Read the model definition and answer for the solid it produces. Units are mm, in the model's axes. A direction names the side the tool comes from. Coordinates: 2 decimals unless noted, no trailing zeros. Order: outer loops, then holes, each group sorted by start corner. A loop starts at its lowest first (then second) coordinate and runs counter-clockwise, first axis right, second up.
Autodesk Inventor part; units mm, degrees
ref_plane "YZ Plane" through (0, 0, 0) normal (1, 0, 0) x (0, 1, 0)
ref_plane "XZ Plane" through (0, 0, 0) normal (0, 1, 0) x (-1, 0, 0)
ref_plane "XY Plane" through (0, 0, 0) normal (0, 0, 1) x (1, 0, 0)
sketch "Sketch1" plane through (0, 0, 0) normal (1, 0, 0) x (0, 1, 0)
  line L0 (0, 0) -> (24, 0)
  line L1 (24, 0) -> (0, 89.5692)
  line L2 (0, 89.5692) -> (0, 0)
  line L3 (24, 0) -> (30, 0)
  line L4 (7.8518, 60.2659) -> (13.6473, 61.8188)
  line L5 (30, 0) -> (0, 113.0916)
  line L6 (0, 113.0916) -> (0, 89.5692)
  point P0 (0, 23.8051)
  point P1 (17.3305, 0)
  point P2 (0, 30.632)
  dimension "d0" = 24
  dimension "d1" = 75
  dimension "d2" = 6
  dimension "d3" = 6
  dimension "d4" = 90
extrude "Extrusion1" add sketch "Sketch1" along normal blind 40
sketch "Sketch5" plane through (0, 0, 0) normal (0, 0, -1) x (-1, 0, 0)
  line L0 (0, 0) -> (0, 30)
  line L1 (-40, 0) -> (-4, 0)
  line L2 (-4, 0) -> (-4, 14)
  line L3 (-4, 14) -> (-40, 14)
  line L4 (-40, 14) -> (-40, 0)
  point P0 (0, 18)
  dimension "d24" = 36
  dimension "d25" = 14
extrude "Extrusion2" cut sketch "Sketch5" against normal blind 52.575
sketch "Sketch7" plane through (4, 14, 0) normal (0, -1, 0) x (1, 0, 0)
  line L0 (0, 0) -> (0, 52.575)
  line L1 (36, 52.575) -> (0, 0)
  line L2 (0, 0) -> (0, 3.8616)
  line L3 (0, 3.8616) -> (33.3558, 52.575)
  line L4 (36, 52.575) -> (0, 52.575)
  line L5 (33.3558, 52.575) -> (36, 52.575)
  point P0 (-4, 0)
extrude "Extrusion4" add sketch "Sketch7" along normal blind 14 contours L0 L3 L4 L1
sketch "Sketch8" plane through (0, 0, 0) normal (0, -1, 0) x (1, 0, 0)
  line L0 (36.9948, 58.9837) -> (3.2686, 58.9837)
  line L1 (3.2686, 58.9837) -> (3.2686, 93.3042)
  line L2 (3.2686, 93.3042) -> (36.9948, 93.3042)
  line L3 (36.9948, 93.3042) -> (36.9948, 58.9837)
  point P0 (0, 0)
extrude "Extrusion5" cut sketch "Sketch8" against normal blind 3.4625
sketch "Sketch9" plane through (0, 3.4625, 0) normal (0, -1, 0) x (1, 0, 0)
  line L0 (36.9948, 58.9837) -> (3.2686, 58.9837)
  line L1 (3.2686, 58.9837) -> (3.2686, 93.3042)
  line L2 (36.9948, 58.9837) -> (3.2686, 58.9837)
  line L3 (3.2686, 58.9837) -> (3.2686, 72.9495)
  line L4 (3.2686, 72.9495) -> (36.9948, 72.9495)
  line L5 (36.9948, 72.9495) -> (36.9948, 58.9837)
  point P0 (0, 0)
extrude "Extrusion6" cut sketch "Sketch9" against normal blind 6.0625
sketch "Sketch10" plane through (0, 0, 0) normal (0, 0, -1) x (-1, 0, 0)
  line L0 (-40, 30) -> (-40, 0)
  line L1 (0, 30) -> (0, 0)
  line L2 (-40, 27) -> (0, 27)
  line L3 (0, 27) -> (0, 21)
  line L4 (0, 21) -> (-40, 21)
  line L5 (-40, 21) -> (-40, 27)
  line L6 (0, 30) -> (-40, 30)
  dimension "d35" = 6
  dimension "d36" = 3
extrude "Extrusion7" add sketch "Sketch10" along normal blind 6 contours L2 L1 L4 L0
properties part number "RAMP"
1) Flat-ended cylindrical pins translate along their axes: pin 1 Ø18 at (x, z) = (21.5, 34) entering from -Y; pin 2 Ø2.5 at (x, y) = (29.5, 29) entering from -Z; pin 3 Ø4 at (x, z) = (27.5, 66.5) entering from -Y (3 decimals); pin 4 Ø4 at (x, y) = (19.5, 1.5) entering from -Z. Find the tip coordinate at first contact, or state that the pin passes through.
A:
pin 1: stops at y = 0
pin 2: stops at z = 0
pin 3: stops at y = 9.525
pin 4: stops at z = 19.72
2) A cutting plane is placed at D-D, the plane y = 11.5. Determine the outline of the cut face in (x, z) (3 decimals).
A:
outline: (0, 0) - (4, 0) - (40, 52.575) - (40, 69.74) - (0, 69.74) - close; hole (4, 3.862) - (37.356, 52.575) - (4, 52.575) - close
3) A cutting plane is placed at A-A, the plane y = 6.75. Determine the outline of the cut face in (x, z) (1 decimal), and give its area (3 significant figures).
A:
outline: (0, 0) - (4, 0) - (40, 52.6) - (40, 87.6) - (0, 87.6) - close; hole (3.3, 59) - (37, 59) - (37, 72.9) - (3.3, 72.9) - close; hole (4, 3.9) - (37.4, 52.6) - (4, 52.6) - close
area: 1,280 mm2
4) Which of the six approach directions +Z, -Z, +X, -X, +Y, -Y give full straight-line access (tool end or side, diameter ignored) to faces 1 (the flat face through (20, 21, -3)), 2 (the flat face through (20, 27, -3)), 3 (the flat face through (4, 7, 28))?
A:
face 1: -Z, +X, -X, -Y
face 2: -Z, +X, -X, +Y
face 3: -Y
5) Determine the mould class of faces 4 (the flat face through (22.252, 7.098, 26.656)), 5 (the flat face through (15, 15, 0)), 6 (the flat face through (20.444, 7.098, 27.877)) for opening direction X: pulls with the +X half, pulls with the -X half, needs draft (parallel to the pull), parting line crosses it, or undercut.
A:
face 4: pulls with the +X half
face 5: needs draft
face 6: undercut
6) Straight lines are drawn through the part: line 1 (X direction, y = 2.75, z = 84.5); line 2 (Y direction, x = 19.5, z = 98); line 3 (X direction, y = 4.75, z = 8). For each, find the intervals that lie inside material, in ascending order.
A:
line 1: x = 0 to 3.27, 36.99 to 40
line 2: y = 0 to 4
line 3: x = 0 to 4, 6.83 to 9.48
7) A cutting plane is placed at B-B, the plane x = 25. Determine the outline of the cut face in (y, z) (1 decimal), and give its area (3 significant figures).
A:
outline: (0, 30.7) - (14, 30.7) - (14, 0) - (21, 0) - (21, -6) - (27, -6) - (27, 0) - (30, 0) - (0, 113.1) - (0, 93.3) - (3.5, 93.3) - (3.5, 72.9) - (9.5, 72.9) - (9.5, 59) - (0, 59) - (0, 52.6) - (14, 52.6) - (14, 34.5) - (0, 34.5) - close
area: 847 mm2
8) A cutting plane is placed at C-C, the plane z = 63. Determine the outline of the cut face in (x, y) (3 decimals).
A:
outline: (0, 0) - (3.269, 0) - (3.269, 9.525) - (36.995, 9.525) - (36.995, 0) - (40, 0) - (40, 13.288) - (0, 13.288) - close
